from build123d import *

# Parameters (mm, degrees)
F1_DEPTH   = 25.4
F2_R       = 12.7
F3_DEPTH   = 25.401
F1_FACE1_W = 50.8
F1_FACE1_H = 25.4
F4_ANGLE   = 115


with BuildPart() as f1:
    # F0 (on Front) → F1 (new body)
    with BuildSketch(Plane.XZ):
        Polygon((0, 50.8), (-50.8, 50.8), (-50.8, -16.5059205686), (0, 0), align=None)
    extrude(amount=F1_DEPTH)

    # F2 (on face) → F3 (cut, through all)
    with BuildSketch(Plane.XZ.offset(25.4)):
        with Locations((-25.4, 25.4)):
            Circle(F2_R)
    extrude(amount=-F3_DEPTH, mode=Mode.SUBTRACT)

    # F1_face1 (on face) → F4 (revolve)
    with BuildSketch(Plane(origin=(-25.4, -12.7, 50.8), x_dir=(1, 0, 0), z_dir=(0, 0, 1))):
        Rectangle(F1_FACE1_W, F1_FACE1_H)
    revolve(axis=Axis((0, -12.7, 50.8), (0, 1, 0)), revolution_arc=F4_ANGLE)


solid = f1.part
Geometry: final body of the model. Coordinates: model frame, mm. A direction names the side the tool comes from. Coordinates: 2 decimals unless noted, no trailing zeros. Order: outer loops, then holes, each group sorted by start corner. A loop starts at its lowest first (then second) coordinate and runs counter-clockwise, first axis right, second up. Notation, with made-up numbers: (76.5, 64.5) - (99.5, 64.5) arc R22 ccw to (99.5, 99.5) - close; hole circle Ø2 at (89, 73.5). An arc over 180 degrees is marked (long way). Use one line per item in the form item = value.
1) Section D-D (x = 17). Return loops of the section in (y, z).
Solutions:
outline = (-25.4, 87.26) - (0, 87.26) - (0, 98.67) - (-25.4, 98.67) - close
2) Set-up query: faces 1 (the face through (-50.8, -13, 18)), 2 (the face through (0, -13, 25)). Return all of +Z, -Z, +X, -X, +Y, -Y with unobstructed straight access to the full face (end or side cutting, diameter ignored); none if empty.
Solutions:
face_1 = +Z, -Z, -X, +Y, -Y
face_2 = -Z, +X, +Y, -Y
3) Pin query (flat end, axial travel): pin 1 (2 mm diameter, centred on x = -14.5, y = -11, fed in from -Z); pin 2 (7.5 mm diameter, centred on y = -18.5, z = 18.5, fed in from +X); pin 3 (1.5 mm diameter, centred on x = -39.5, z = 63, fed in from +Y); pin 4 (1 mm diameter, centred on x = -17, y = -16.5, fed in from -Z). Return the tip coordinate at first contact, or that it passes through.
Solutions:
pin_1 = -5.04
pin_2 = 0
pin_3 = 0
pin_4 = -5.69
4) Section C-C (y = -22). Return loops of the section in (x, z), then the cut area to 3 significant figures.
Solutions:
outline = (-50.8, -16.51) - (0, 0) - (0, 50.8) - (21.47, 96.84) arc R50.8 ccw to (-50.8, 50.8) - close; hole circle Ø25.4 at (-25.4, 25.4)
area = 5,080 mm^2
5) Section A-A (z = 25.4). Return loops of the section in (x, y), then the cut area to 3 significant figures.
Solutions:
outline = (-50.8, -25.4) - (-38.1, -25.4) - (-38.1, 0) - (-50.8, 0) - close; (-12.7, -25.4) - (0, -25.4) - (0, 0) - (-12.7, 0) - close
area = 645 mm^2
6) Mould query, pull axis Z, two halves, no side actions, for faces 3 (the face through (-22, -25.4, 56)), 4 (the face through (-25.76, -12.52, -8.37)), 5 (the face through (-18.573, -12.878, 36.109)). Classes: +Z half, -Z half, draft (parallel to the pull), parting line (faces both ways), or undercut.
Solutions:
face_3 = draft
face_4 = -Z half
face_5 = undercut
7) Ray query, L1, parallel to Z at x = -33, y = -18.5; L2, parallel to Z at x = -31, y = -11.75; L3, parallel to X at y = -2.25, z = 11. Return the intervals inside material, ascending.
Solutions:
L1 = -10.72 to 15.23, 35.57 to 89.42
L2 = -10.07 to 14, 36.8 to 91.04
L3 = -50.8 to 0
8) Section B-B (x = -25.4). Return loops of the section in (y, z), then the cut area to 3 significant figures.
Solutions:
outline = (-25.4, -8.25) - (0, -8.25) - (0, 12.7) - (-25.4, 12.7) - close; (-25.4, 38.1) - (0, 38.1) - (0, 94.79) - (-25.4, 94.79) - close
area = 1,970 mm^2
